Geometry: see drawing. Coordinates: mm, zero at the bounding-box minimum. A direction names the side the tool comes from. Give positions to 0.01 mm unless a question says otherwise; leave off trailing zeros. Loops run counter-clockwise (first coordinate to the right, second up) from the corner with the lowest first, then second, coordinate; pieces in that order, holes last. Notation, with made-up numbers: (-2, 37) - (52, 37) arc R13 cw to (52, 50) - close; hole circle Ø11 at (30, 17). An arc over 180 degrees is marked (long way). Use one line per item in the form item = value.
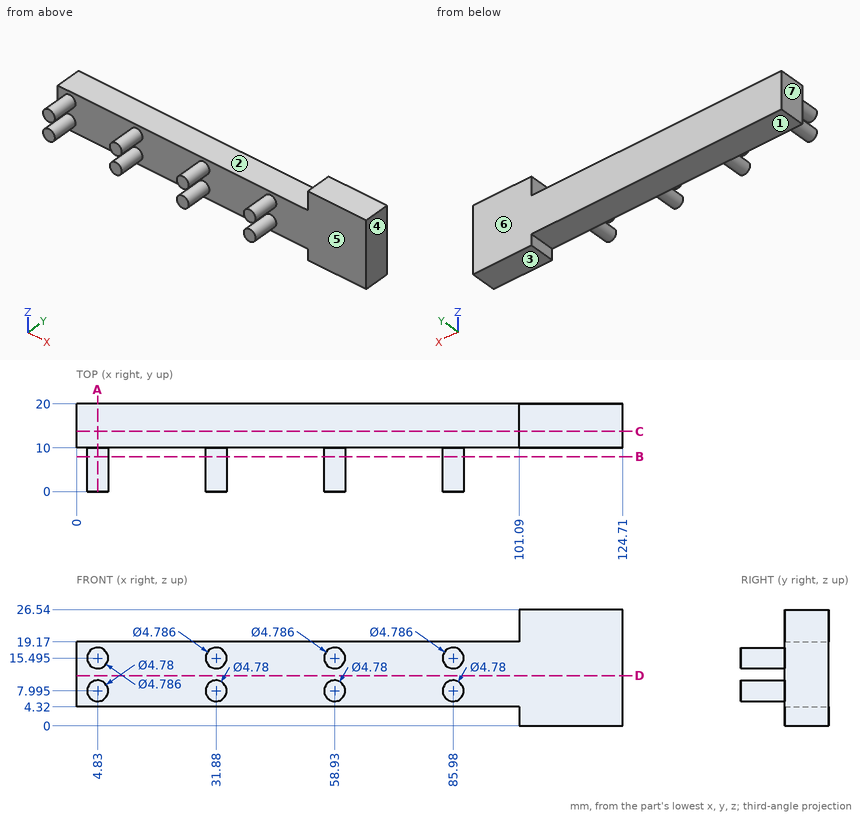
(1) Pull-direction query (X, two-part tool) for the marked faces 4, 5, 6 and 7; classes: released by +X, released by -X, zero draft, split by the parting line, or undercut.
Solution:
face_4 = released by +X
face_5 = undercut
face_6 = zero draft
face_7 = released by -X
(2) Cut plane A-A (x = 4.83). Return the cut outline in (y, z) (3 decimals).
Solution:
outline = (0, 5.605) - (10, 5.605) - (10, 4.32) - (20, 4.32) - (20, 19.17) - (10, 19.17) - (10, 17.888) - (0, 17.888) - (0, 13.102) - (10, 13.102) - (10, 10.385) - (0, 10.385) - close
(3) Access query for the marked faces 1, 2 and 3. Directions: +Z, -Z, +X, -X, +Y, -Y. A direction counts if a zero-diameter tool reaches every point of the face in a straight line with its end or side. Return the directions, or none.
Solution:
face_1 = -Z, -X, +Y, -Y
face_2 = +Z, -X, +Y, -Y
face_3 = -Z, +X, -X, +Y, -Y
(4) Pin query (flat end, axial travel): P1, Ø1.5, axis at x = 72.5, y = 18, coming from the -Z side; P2, Ø3, axis at y = 2.5, z = 12, coming from the +X side; P3, Ø6, axis at x = 44.5, y = 12.5, coming from the +Z side. Return the tip coordinate at first contact, or that it passes through.
Solution:
P1 = 4.32
P2 = 87.3
P3 = 19.17
(5) Cut plane C-C (y = 13.75). Return the cut outline in (x, z).
Solution:
outline = (0, 4.32) - (101.09, 4.32) - (101.09, 0) - (124.71, 0) - (124.71, 26.54) - (101.09, 26.54) - (101.09, 19.17) - (0, 19.17) - close
(6) Cut plane B-B (y = 8). Return the cut outline in (x, z) (3 decimals), plus the area to 3 significant figures.
Solution:
outline = circle Ø4.786 at (4.83, 15.495); circle Ø4.78 at (4.83, 7.995); circle Ø4.786 at (31.88, 15.495); circle Ø4.78 at (31.88, 7.995); circle Ø4.786 at (58.93, 15.495); circle Ø4.78 at (58.93, 7.995); circle Ø4.786 at (85.98, 15.495); circle Ø4.78 at (85.98, 7.995)
area = 144 mm2
(7) Material intervals for L1, parallel to X at y = 4.25, z = 16.5; L2, parallel to Z at x = 51.5, y = 11.25; L3, parallel to Y at x = 101, z = 6.5, sorted ascending. Write a range as from..to.
Solution:
L1 = 2.66..7, 29.71..34.05, 56.76..61.1, 83.81..88.15
L2 = 4.32..19.17
L3 = 10..20
(8) Cut plane D-D (z = 11.5). Return the cut outline in (x, y).
Solution:
outline = (0, 10) - (124.71, 10) - (124.71, 20) - (0, 20) - close
